Autodesk Inventor part; units mm, degrees
ref_plane "YZ Plane" through (0, 0, 0) normal (1, 0, 0) x (0, 1, 0)
ref_plane "XZ Plane" through (0, 0, 0) normal (0, 1, 0) x (-1, 0, 0)
ref_plane "XY Plane" through (0, 0, 0) normal (0, 0, 1) x (1, 0, 0)
sketch "Sketch1" plane through (0, 0, 0) normal (0, 0, 1) x (1, 0, 0)
  line L0 (-38.8739, 0) -> (58.9391, 0) construction
  line L1 (0, -36.2399) -> (0, 43.1348) construction
  line L2 (0, 0) -> (31.7956, 31.7956) construction
  line L3 (0, 0) -> (44.9658, 0) construction
  line L4 (0, 24.9006) -> (16.8, 24.9006)
  line L5 (16.8, 24.9006) -> (16.8, 21.2406)
  line L6 (16.8, 21.2406) -> (19.0203, 19.0203)
  line L7 (24.9006, 0) -> (24.9006, 16.8)
  line L8 (24.9006, 16.8) -> (21.2406, 16.8)
  line L9 (21.2406, 16.8) -> (19.0203, 19.0203)
  line L10 (0, 24.9006) -> (-16.8, 24.9006)
  line L11 (-16.8, 24.9006) -> (-16.8, 21.2406)
  line L12 (-16.8, 21.2406) -> (-19.0203, 19.0203)
  line L13 (-24.9006, 0) -> (-24.9006, 16.8)
  line L14 (-24.9006, 16.8) -> (-21.2406, 16.8)
  line L15 (-21.2406, 16.8) -> (-19.0203, 19.0203)
  line L16 (0, -24.9006) -> (16.8, -24.9006)
  line L17 (16.8, -24.9006) -> (16.8, -21.2406)
  line L18 (16.8, -21.2406) -> (19.0203, -19.0203)
  line L19 (24.9006, 0) -> (24.9006, -16.8)
  line L20 (24.9006, -16.8) -> (21.2406, -16.8)
  line L21 (21.2406, -16.8) -> (19.0203, -19.0203)
  line L22 (0, -24.9006) -> (-16.8, -24.9006)
  line L23 (-16.8, -24.9006) -> (-16.8, -21.2406)
  line L24 (-16.8, -21.2406) -> (-19.0203, -19.0203)
  line L25 (-24.9006, 0) -> (-24.9006, -16.8)
  line L26 (-24.9006, -16.8) -> (-21.2406, -16.8)
  line L27 (-21.2406, -16.8) -> (-19.0203, -19.0203)
  circle A0 centre (0, 0) radius 14
  dimension "d0" = 45
  dimension "d1" = 16.8
  dimension "d2" = 3.66
  dimension "d3" = 3.14
  dimension "d4" = 28
extrude "Extrusion1" add sketch "Sketch1" along normal blind 5
sketch "Sketch2" plane through (0, 0, 5) normal (0, 0, 1) x (1, 0, 0)
  circle A0 centre (0, 0) radius 14 construction
  line L0 (16.8, 24.9006) -> (-16.8, 24.9006) construction
  line L1 (-16.8, 24.9006) -> (-16.8, 21.2406) construction
  line L2 (-16.8, 21.2406) -> (-21.2406, 16.8) construction
  line L3 (-21.2406, 16.8) -> (-24.9006, 16.8) construction
  line L4 (-24.9006, 16.8) -> (-24.9006, -16.8) construction
  line L5 (-24.9006, -16.8) -> (-21.2406, -16.8) construction
  line L6 (-21.2406, -16.8) -> (-16.8, -21.2406) construction
  line L7 (-16.8, -21.2406) -> (-16.8, -24.9006) construction
  line L8 (-16.8, -24.9006) -> (16.8, -24.9006) construction
  line L9 (16.8, -24.9006) -> (16.8, -21.2406) construction
  line L10 (16.8, -21.2406) -> (21.2406, -16.8) construction
  line L11 (21.2406, -16.8) -> (24.9006, -16.8) construction
  line L12 (24.9006, -16.8) -> (24.9006, 16.8) construction
  line L13 (24.9006, 16.8) -> (21.2406, 16.8) construction
  line L14 (21.2406, 16.8) -> (16.8, 21.2406) construction
  line L15 (16.8, 21.2406) -> (16.8, 24.9006) construction
  line L16 (-34.8609, 0) -> (34.8609, 0) construction
  line L17 (0, -34.8609) -> (0, 34.8609) construction
  circle A1 centre (13, -13) radius 2.5
  circle A2 centre (-13, -13) radius 2.5
  dimension "d7" = 5
  dimension "d8" = 13
  dimension "d9" = 13
extrude "Extrusion2" [suppressed]
sketch "Sketch3" plane through (0, 0, 0) normal (1, 0, 0) x (0, 1, 0)
  line L0 (-14, 5) -> (14, 5) construction
  line L1 (24.9006, 5) -> (21.2406, 5) construction
  line L2 (21.2406, 5) -> (16.8, 5) construction
  line L3 (16.8, 5) -> (-16.8, 5) construction
  line L4 (-16.8, 5) -> (-21.2406, 5) construction
  line L5 (-21.2406, 5) -> (-24.9006, 5) construction
  line L6 (-24.9006, 5) -> (-21.2406, 5) construction
  line L7 (-21.2406, 5) -> (-16.8, 5) construction
  line L8 (-16.8, 5) -> (16.8, 5) construction
  line L9 (16.8, 5) -> (21.2406, 5) construction
  line L10 (21.2406, 5) -> (24.9006, 5) construction
  line L11 (24.9006, 0) -> (21.2406, 0) construction
  line L12 (24.9006, 0) -> (24.9006, 5) construction
  line L13 (21.2406, 5) -> (24.9006, 5) construction
  line L14 (21.2406, 0) -> (21.2406, 5) construction
  line L15 (21.2406, 0) -> (16.8, 0) construction
  line L16 (21.2406, 0) -> (21.2406, 5) construction
  line L17 (16.8, 5) -> (21.2406, 5) construction
  line L18 (16.8, 0) -> (16.8, 5) construction
  line L19 (16.8, 0) -> (-16.8, 0) construction
  line L20 (16.8, 0) -> (16.8, 5) construction
  line L21 (-16.8, 5) -> (16.8, 5) construction
  line L22 (-16.8, 0) -> (-16.8, 5) construction
  line L23 (-16.8, 0) -> (-21.2406, 0) construction
  line L24 (-16.8, 0) -> (-16.8, 5) construction
  line L25 (-21.2406, 5) -> (-16.8, 5) construction
  line L26 (-21.2406, 0) -> (-21.2406, 5) construction
  line L27 (-21.2406, 0) -> (-24.9006, 0) construction
  line L28 (-21.2406, 0) -> (-21.2406, 5) construction
  line L29 (-24.9006, 5) -> (-21.2406, 5) construction
  line L30 (-24.9006, 0) -> (-24.9006, 5) construction
  line L31 (-14, 5) -> (14, 5) construction
  line L32 (14, 0) -> (-14, 0) construction
  line L33 (16.8, 5) -> (-16.8, 5)
  arc A0 (0, -9) -> (14, 5) centre (0, 5) ccw
  line L34 (0, -16.0037) -> (0, 8.5006) construction
  arc A1 (0, -11) -> (16, 5) centre (0, 5) ccw
  line L35 (0, -9) -> (0, -11)
  line L36 (16, 5) -> (14, 5)
revolve "Revolution1" add sketch "Sketch3" angle 360 about axis through (0, 0, -10) along (0, 0, 1)
sketch "Skizze4" plane through (0, 0, 5) normal (0, 0, 1) x (1, 0, 0)
  circle A0 centre (0, 0) radius 14 construction
  line L0 (16.8, 24.9006) -> (-16.8, 24.9006) construction
  line L1 (-16.8, 24.9006) -> (-16.8, 21.2406)
  line L2 (-16.8, 21.2406) -> (-21.2406, 16.8)
  line L3 (-21.2406, 16.8) -> (-24.9006, 16.8)
  line L4 (-24.9006, 16.8) -> (-24.9006, -16.8) construction
  line L5 (-24.9006, -16.8) -> (-21.2406, -16.8)
  line L6 (-21.2406, -16.8) -> (-16.8, -21.2406)
  line L7 (-16.8, -21.2406) -> (-16.8, -24.9006)
  line L8 (-16.8, -24.9006) -> (16.8, -24.9006) construction
  line L9 (16.8, -24.9006) -> (16.8, -21.2406)
  line L10 (16.8, -21.2406) -> (21.2406, -16.8)
  line L11 (21.2406, -16.8) -> (24.9006, -16.8)
  line L12 (24.9006, -16.8) -> (24.9006, 16.8) construction
  line L13 (24.9006, 16.8) -> (21.2406, 16.8)
  line L14 (21.2406, 16.8) -> (16.8, 21.2406)
  line L15 (16.8, 21.2406) -> (16.8, 24.9006)
  line L16 (-16.9, 25.0006) -> (16.9, 25.0006) construction
  line L17 (16.9, 25.0006) -> (16.9, 21.2821)
  line L18 (16.9, 21.2821) -> (21.2821, 16.9)
  line L19 (21.2821, 16.9) -> (25.0006, 16.9)
  line L20 (25.0006, 16.9) -> (25.0006, -16.9) construction
  line L21 (25.0006, -16.9) -> (21.2821, -16.9)
  line L22 (21.2821, -16.9) -> (16.9, -21.2821)
  line L23 (16.9, -21.2821) -> (16.9, -25.0006)
  line L24 (16.9, -25.0006) -> (-16.9, -25.0006) construction
  line L25 (-16.9, -25.0006) -> (-16.9, -21.2821)
  line L26 (-16.9, -21.2821) -> (-21.2821, -16.9)
  line L27 (-21.2821, -16.9) -> (-25.0006, -16.9)
  line L28 (-25.0006, -16.9) -> (-25.0006, 16.9) construction
  line L29 (-25.0006, 16.9) -> (-21.2821, 16.9)
  line L30 (-21.2821, 16.9) -> (-16.9, 21.2821)
  line L31 (-16.9, 21.2821) -> (-16.9, 25.0006)
  line L32 (-24.9006, 16.8) -> (-24.9006, 16.9)
  line L33 (16.8, 24.9006) -> (-16.8, 24.9006)
  line L34 (-16.8, 24.9006) -> (-16.9, 24.9006)
  line L35 (16.8, 24.9006) -> (16.9, 24.9006)
  line L36 (24.9006, -16.8) -> (24.9006, 16.8)
  line L37 (24.9006, 16.8) -> (24.9006, 16.9)
  line L38 (24.9006, -16.8) -> (24.9006, -16.9)
  line L39 (16.8, -24.9006) -> (16.8, -21.2406)
  line L40 (16.8, -24.9006) -> (16.9, -24.9006)
  line L41 (-16.8, -24.9006) -> (-16.9, -24.9006)
  line L42 (-24.9006, -16.8) -> (-24.9006, 16.8)
  line L43 (-24.9006, -16.8) -> (-24.9006, -16.9)
  dimension "d15" = 0.1
extrude "IM_offset" add sketch "Skizze4" against normal up to surface (5 mm away)
equation "\"d9\" = d8"
properties part number "20_Cube_Insert_Eye_v3"
CAD build for the part. Positions are in the model's coordinates, mm. A direction names the side the tool comes from. Coordinates: 2 decimals unless noted, no trailing zeros. Order: outer loops, then holes, each group sorted by start corner. A loop starts at its lowest first (then second) coordinate and runs counter-clockwise, first axis right, second up.
(1) Saw through at A-A, the plane x = 5. Write the cut outline in (y, z), and give its area (3 significant figures).
Solution:
outline: (-24.9, 0) - (-14.35, 0) arc R15.2 ccw to (14.35, 0) - (24.9, 0) - (24.9, 5) - (13.08, 5) arc R13.08 cw to (-13.08, 5) - (-24.9, 5) - close
area: 194 mm2
(2) Saw through at B-B, the plane y = 2.5. Write the cut outline in (x, z).
Solution:
outline: (-24.9, 0) - (-14.99, 0) arc R15.8 ccw to (14.99, 0) - (24.9, 0) - (24.9, 5) - (13.77, 5) arc R13.77 cw to (-13.77, 5) - (-24.9, 5) - close
(3) Saw through at C-C, the plane z = -7.75. Write the cut outline in (x, y).
Solution:
outline: circle Ø19.33 at (0, 0); hole circle Ø11.57 at (0, 0)
(4) Mould opens along X. For faces 6 (the face through (-11, -11, 0)), 7 (the face through (-24.901, 0, 2)), 8 (the face through (16.9, -23, 3)) say: released by +X, released by -X, zero draft, split by the parting line, or undercut.
Solution:
face 6: zero draft
face 7: released by -X
face 8: released by +X
(5) Which spindle directions (+Z, -Z, +X, -X, +Y, -Y) get a long thin tool onto all of the face, cutting with end or side? Do faces 1 (the face through (23, -16.9, 3)), 2 (the face through (-23, 16.9, 3)), 3 (the face through (16.9, 23, 3)), 4 (the face through (-23, -16.9, 3)), 5 (the face through (11, -11, 5)). Say none if no direction does.
Solution:
face 1: +Z, -Z, +X, -Y
face 2: +Z, -Z, -X, +Y
face 3: +Z, -Z, +X, +Y
face 4: +Z, -Z, -X, -Y
face 5: +Z, +X, -X, +Y, -Y
(6) Saw through at D-D, the plane y = 22. Write the cut outline in (x, z).
Solution:
outline: (-16.9, 0) - (16.9, 0) - (16.9, 5) - (-16.9, 5) - close
(7) Pin check, flat tips, straight feed: pin 1 Ø1.8 at (x, z) = (-22, 3) entering from +Y; pin 2 Ø3 at (x, z) = (22.5, 1.5) entering from -Y; pin 3 Ø1.5 at (x, z) = (3.5, -5.5) entering from -Y. Stop position of each tip, or through.
Solution:
pin 1: stops at y = 17.08
pin 2: stops at y = -17.18
pin 3: stops at y = -12.23
(8) Drill centre lines: L1, parallel to Z at x = 1.5, y = -20; L2, parallel to Y at x = -2.5, z = -5.75; L3, parallel to Y at x = 23.5, z = 2.25. Where is each one in solid material? Low to high.
Solution:
L1: z = 0 to 5
L2: y = -11.58 to -8.61, 8.61 to 11.58
L3: y = -16.9 to 16.9
